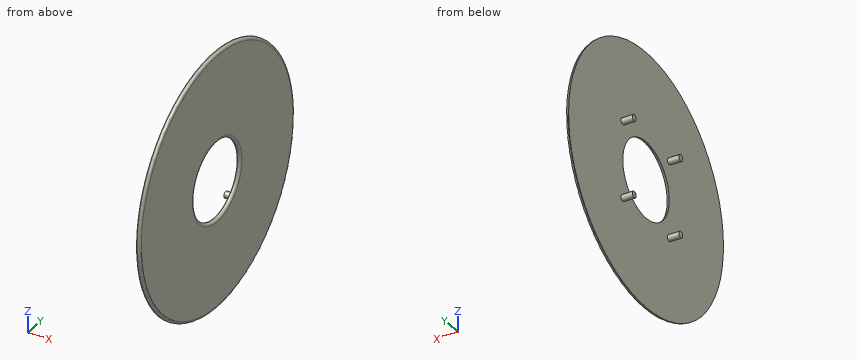
```python
from build123d import *

# Parameters (mm, degrees)
SKETCH1_R           = 25.4
SKETCH1_R_2         = 7.62
BOSS_EXTRUDE1_DEPTH = 0.635
FILLET1_R           = 0.508
SKETCH2_R           = 0.635
BOSS_EXTRUDE2_DEPTH = 2.286


with BuildPart() as part:
    # Sketch1 → Boss-Extrude1 (new body)
    with BuildSketch(Plane(origin=(0, 0, 0), x_dir=(0, 0, -1), z_dir=(1, 0, 0))):
        Circle(SKETCH1_R)
        Circle(SKETCH1_R_2, mode=Mode.SUBTRACT)
    extrude(amount=BOSS_EXTRUDE1_DEPTH)

    # Fillet1
    fillet1_edges = [part.edges().sort_by_distance(p)[0] for p in [
        (0.635, 0, 25.4),
        (0.635, 0, 7.62),
    ]]
    fillet(fillet1_edges, radius=FILLET1_R)

    # Sketch2 → Boss-Extrude2 (add)
    with BuildSketch(Plane.ZY):
        with Locations((-7.633217703, 7.633217703)):
            Circle(SKETCH2_R)
        with Locations((7.633217703, 7.633217703)):
            Circle(SKETCH2_R)
        with Locations((7.633217703, -7.633217703)):
            Circle(SKETCH2_R)
        with Locations((-7.633217703, -7.633217703)):
            Circle(SKETCH2_R)
    extrude(amount=BOSS_EXTRUDE2_DEPTH)


solid = part.part
```
Source: CAD feature listing. Evaluate the final solid. Frame: model axes, mm. Coordinates: 2 decimals unless noted, no trailing zeros. Loops run counter-clockwise (first coordinate to the right, second up) from the corner with the lowest first, then second, coordinate; pieces in that order, holes last. Notation, with made-up numbers: (-10, 2) -> (16, 2) arc R15 cw to (16, 15) -> close; hole circle Ø1 at (16.25, -29). An arc over 180 degrees is marked (long way). One line per item, written item: value. Start each with the question number.
Q1. Section query A-A, the plane y = 0. Return the cut outline in (x, z) (3 decimals).
Q2. Line query: line 1 along Y through (x, z) = (0.1, 0); line 2 along X through (y, z) = (-14, -15) (3 decimals); line 3 along Z through (x, y) = (0.3, -19). Output: solid intervals per line, ascending.
Q3. Section query C-C, the plane x = -1.4. Return the cut outline in (y, z) (3 decimals), and give its area (3 significant figures).
Q4. Contact query for a flat-ended pin moving along its axis: P1, Ø6, axis at y = 13.5, z = 17, coming from the -X side. Output: stop coordinate, or through.
Results:
1. outline: (0, -25.4) -> (0.127, -25.4) arc R0.508 ccw to (0.635, -24.892) -> (0.635, -8.128) arc R0.508 ccw to (0.127, -7.62) -> (0, -7.62) -> close; (0, 7.62) -> (0.127, 7.62) arc R0.508 ccw to (0.635, 8.128) -> (0.635, 24.892) arc R0.508 ccw to (0.127, 25.4) -> (0, 25.4) -> close
2. line 1: -25.4 to -7.62, 7.62 to 25.4
2. line 2: 0 to 0.635
2. line 3: -16.81 to 16.81
3. outline: circle Ø1.27 at (-7.633, -7.633); circle Ø1.27 at (-7.633, 7.633); circle Ø1.27 at (7.633, -7.633); circle Ø1.27 at (7.633, 7.633)
3. area: 5.07 mm^2
4. P1: x = 0
